Design review of the part built by this model. Coordinates are the model's own, in mm. A direction names the side the tool comes from. Coordinates: 2 decimals unless noted, no trailing zeros. Loops run counter-clockwise (first coordinate to the right, second up) from the corner with the lowest first, then second, coordinate; pieces in that order, holes last.
from build123d import *

# Parameters (mm, degrees)
SKETCH1_W           = 66
SKETCH1_H           = 95
SKETCH1_R           = 20
BOSS_EXTRUDE1_DEPTH = 12
BOSS_EXTRUDE3_DEPTH = 12
SKETCH6_R           = 6
CUT_EXTRUDE2_DEPTH  = 6
CHAMFER1_SIZE       = 20
CUT_EXTRUDE3_REACH  = 91.828
SKETCH7_R           = 3
SKETCH7_R_2         = 5
SKETCH9_R           = 3
CUT_EXTRUDE5_DEPTH  = 25
CUT_EXTRUDE6_REACH  = 91.828
SKETCH10_R          = 2.5
CUT_EXTRUDE7_DEPTH  = 4


with BuildPart() as part:
    # Sketch1 → Boss-Extrude1 (new body)
    with BuildSketch(Plane(origin=(0, 0, 0), x_dir=(1, 0, 0), z_dir=(0, 1, 0))):
        with Locations((0, -22.5)):
            Rectangle(SKETCH1_W, SKETCH1_H)
        with Locations(Location((0, -30, 0), (0, 0, 270))):
            Circle(SKETCH1_R, mode=Mode.SUBTRACT)
    extrude(amount=BOSS_EXTRUDE1_DEPTH)

    # Sketch3 → Boss-Extrude3 (add)
    with BuildSketch(Plane(origin=(0, 12, 0), x_dir=(1, 0, 0), z_dir=(0, 1, 0))):
        Polygon((55, 7), (43, 7), (43, -11), (55, -11), (55, -70), (33, -70), (33, 25), (55, 25), align=None)
    boss_extrude3 = extrude(amount=-BOSS_EXTRUDE3_DEPTH)

    # Mirror1: Boss-Extrude3 across plane
    add(boss_extrude3.mirror(Plane(origin=(0, 0, 0), x_dir=(0, 0, 1), z_dir=(1, 0, 0))))

    # Sketch6 → Cut-Extrude2 (cut)
    with BuildSketch(Plane(origin=(0, 12, 0), x_dir=(1, 0, 0), z_dir=(0, 1, 0))):
        with Locations(Location((-28, -51, 0), (0, 0, 270))):
            Circle(SKETCH6_R)
        with Locations(Location((28, -51, 0), (0, 0, 270))):
            Circle(SKETCH6_R)
    extrude(amount=-CUT_EXTRUDE2_DEPTH, mode=Mode.SUBTRACT)

    # Chamfer1
    chamfer1_edges = [part.edges().sort_by_distance(p)[0] for p in [
        (55, 6, 70),
        (-55, 6, 70),
    ]]
    chamfer(chamfer1_edges, length=CHAMFER1_SIZE)

    # Sketch7 → Cut-Extrude3 (cut, up to next)
    with BuildSketch(Plane(origin=(0, 12, 0), x_dir=(1, 0, 0), z_dir=(0, 1, 0)), mode=Mode.PRIVATE) as cut_extrude3_sk1:
        with Locations(Location((-49, 16, 0), (0, 0, 270))):
            Circle(SKETCH7_R)
    cut_extrude3_tool1 = extrude(cut_extrude3_sk1.sketch, amount=-CUT_EXTRUDE3_REACH, mode=Mode.PRIVATE) & part.part
    # Sketch7 → Cut-Extrude3 (cut, up to next)
    with BuildSketch(Plane(origin=(0, 12, 0), x_dir=(1, 0, 0), z_dir=(0, 1, 0)), mode=Mode.PRIVATE) as cut_extrude3_sk2:
        with Locations(Location((-49, -20, 0), (0, 0, 270))):
            Circle(SKETCH7_R)
    cut_extrude3_tool2 = extrude(cut_extrude3_sk2.sketch, amount=-CUT_EXTRUDE3_REACH, mode=Mode.PRIVATE) & part.part
    # Sketch7 → Cut-Extrude3 (cut, up to next)
    with BuildSketch(Plane(origin=(0, 12, 0), x_dir=(1, 0, 0), z_dir=(0, 1, 0)), mode=Mode.PRIVATE) as cut_extrude3_sk3:
        with Locations(Location((-25, -2, 0), (0, 0, 270))):
            Circle(SKETCH7_R_2)
    cut_extrude3_tool3 = extrude(cut_extrude3_sk3.sketch, amount=-CUT_EXTRUDE3_REACH, mode=Mode.PRIVATE) & part.part
    cut_extrude3_1 = cut_extrude3_tool1.solids().sort_by_distance((-49, 12, -16))[0]
    add(cut_extrude3_1, mode=Mode.SUBTRACT)
    cut_extrude3_2 = cut_extrude3_tool2.solids().sort_by_distance((-49, 12, 20))[0]
    add(cut_extrude3_2, mode=Mode.SUBTRACT)
    cut_extrude3_3 = cut_extrude3_tool3.solids().sort_by_distance((-25, 12, 2))[0]
    add(cut_extrude3_3, mode=Mode.SUBTRACT)
    cut_extrude3 = cut_extrude3_1 + cut_extrude3_2 + cut_extrude3_3  # Cut-Extrude3 as one shape, for the pattern or mirror that repeats it

    # Sketch9 → Cut-Extrude5 (cut)
    with BuildSketch(Plane.ZY.offset(43)):
        with Locations((2, 6)):
            Circle(SKETCH9_R)
    cut_extrude5 = extrude(amount=-CUT_EXTRUDE5_DEPTH, mode=Mode.SUBTRACT)

    # Mirror2: Cut-Extrude3, Cut-Extrude5 across plane
    add(cut_extrude3.mirror(Plane(origin=(0, 0, 0), x_dir=(0, 0, 1), z_dir=(1, 0, 0))), mode=Mode.SUBTRACT)
    add(cut_extrude5.mirror(Plane(origin=(0, 0, 0), x_dir=(0, 0, 1), z_dir=(1, 0, 0))), mode=Mode.SUBTRACT)

    # Sketch10 → Cut-Extrude6 (cut, up to next)
    with BuildSketch(Plane.XZ, mode=Mode.PRIVATE) as cut_extrude6_sk1:
        with Locations(Location((0, 63.234018716, 0), (0, 0, 270))):
            Circle(SKETCH10_R)
    cut_extrude6_tool1 = extrude(cut_extrude6_sk1.sketch, amount=-CUT_EXTRUDE6_REACH, mode=Mode.PRIVATE) & part.part
    # Sketch10 → Cut-Extrude6 (cut, up to next)
    with BuildSketch(Plane.XZ, mode=Mode.PRIVATE) as cut_extrude6_sk2:
        with Locations(Location((-33.234018716, 30, 0), (0, 0, 270))):
            Circle(SKETCH10_R)
    cut_extrude6_tool2 = extrude(cut_extrude6_sk2.sketch, amount=-CUT_EXTRUDE6_REACH, mode=Mode.PRIVATE) & part.part
    # Sketch10 → Cut-Extrude6 (cut, up to next)
    with BuildSketch(Plane.XZ, mode=Mode.PRIVATE) as cut_extrude6_sk3:
        with Locations(Location((0, -3.234018716, 0), (0, 0, 270))):
            Circle(SKETCH10_R)
    cut_extrude6_tool3 = extrude(cut_extrude6_sk3.sketch, amount=-CUT_EXTRUDE6_REACH, mode=Mode.PRIVATE) & part.part
    # Sketch10 → Cut-Extrude6 (cut, up to next)
    with BuildSketch(Plane.XZ, mode=Mode.PRIVATE) as cut_extrude6_sk4:
        with Locations(Location((33.234018716, 30, 0), (0, 0, 270))):
            Circle(SKETCH10_R)
    cut_extrude6_tool4 = extrude(cut_extrude6_sk4.sketch, amount=-CUT_EXTRUDE6_REACH, mode=Mode.PRIVATE) & part.part
    add(cut_extrude6_tool1.solids().sort_by_distance((0, 0, 63.234019))[0], mode=Mode.SUBTRACT)
    add(cut_extrude6_tool2.solids().sort_by_distance((-33.234019, 0, 30))[0], mode=Mode.SUBTRACT)
    add(cut_extrude6_tool3.solids().sort_by_distance((0, 0, -3.234019))[0], mode=Mode.SUBTRACT)
    add(cut_extrude6_tool4.solids().sort_by_distance((33.234019, 0, 30))[0], mode=Mode.SUBTRACT)

    # Sketch12 → Cut-Extrude7 (cut)
    with BuildSketch(Plane(origin=(0, 12, 0), x_dir=(1, 0, 0), z_dir=(0, 1, 0))):
        Polygon((3.334261142, -59.954887332), (-1.17268051, -58.706898172), (-4.506941652, -61.986029556), (-3.334261142, -66.5131501), (1.17268051, -67.76113926), (4.506941652, -64.482007876), align=None)
        Polygon((-29.899757573, -33.279131384), (-28.727077064, -28.75201084), (-32.061338206, -25.472879456), (-36.568279858, -26.720868616), (-37.740960368, -31.24798916), (-34.406699225, -34.527120544), align=None)
        Polygon((-3.282764492, -0.096665492), (1.24307489, -1.274280833), (4.525839382, 2.056403375), (3.282764492, 6.564702924), (-1.24307489, 7.742318264), (-4.525839382, 4.411634056), align=None)
        Polygon((29.951254224, -26.669315792), (28.708179334, -31.177615341), (31.990943826, -34.508299548), (36.516783208, -33.330684208), (37.759858098, -28.822384659), (34.477093606, -25.491700452), align=None)
    extrude(amount=-CUT_EXTRUDE7_DEPTH, mode=Mode.SUBTRACT)


solid = part.part
Q1. The part is to be moulded in two halves that separate along Y. For faces 4 (the flat face through (1, 6, -25)), 5 (the cylindrical face through (-19.19, 4.85, 4.77)), 6 (the flat face through (-2, 8, 65)), 7 (the flat face through (18, 6, 2)), say which applies: pulls with the +Y half, pulls with the -Y half, needs draft (parallel to the pull), parting line crosses it, or undercut.
Q2. Take a section at B-B, the plane x = 49. Write out the cut boundary in (y, z), then the cut area to 3 significant figures.
Q3. Take a section at D-D, the plane y = 10.25. Give the number of separate pieces and of enclosed holes in the cut face, then the cut area to 3 significant figures.
Q4. Take a section at A-A, the plane z = -16. Write out the cut boundary in (x, y).
Q5. Machinability: for faces 1 (the flat face through (55, 6, 30)), 2 (the flat face through (-32.18, 10.03, 33.91)), 3 (the flat face through (43, 9, 0)), which of the approach directions +Z, -Z, +X, -X, +Y, -Y give a long, thin tool a straight path to every point of the face, cutting with its end or side? Answer none if there is none.
Q6. For line 1 (X direction, y = 6.75, z = 30); line 2 (X direction, y = 8, z = 55); line 3 (X direction, y = 8, z = -13.5), list the stretches that pass through material, from the lowest coordinate up.
Q7. Take a section at C-C, the plane z = 36.5. Write out the cut boundary in (x, y).
Q8. Clearance check with flat-ended pins moving along their axes: pin 1 Ø5 at (y, z) = (6, 2) entering from -X; pin 2 Ø6 at (x, z) = (29, 53.5) entering from +Y; pin 3 Ø6 at (x, y) = (-40.5, 5) entering from +Z. State where each tip first meets the part, or that it passes through.
Entries:
1. face 4: needs draft
1. face 5: undercut
1. face 6: pulls with the +Y half
1. face 7: undercut
2. outline: (0, -25) - (12, -25) - (12, -19) - (0, -19) - close; (0, -13) - (12, -13) - (12, -7) - (0, -7) - close; (0, 11) - (12, 11) - (12, 17) - (0, 17) - close; (0, 23) - (12, 23) - (12, 56) - (0, 56) - close
2. area: 612 mm2
3. separate pieces: 1
3. enclosed holes: 13
3. area: 7,640 mm2
4. outline: (-55, 0) - (-52, 0) - (-52, 12) - (-55, 12) - close; (-46, 0) - (46, 0) - (46, 12) - (-46, 12) - close; (52, 0) - (55, 0) - (55, 12) - (52, 12) - close
5. face 1: +Z, -Z, +X, +Y, -Y
5. face 2: +Y
5. face 3: +X, +Y, -Y
6. line 1: x = -55 to -35.73, -30.73 to -20, 20 to 30.73, 35.73 to 55
6. line 2: x = -50 to -32.47, -23.53 to 23.53, 32.47 to 50
6. line 3: x = -55 to -50.66, -47.34 to 47.34, 50.66 to 55
7. outline: (-55, 0) - (-18.91, 0) - (-18.91, 12) - (-55, 12) - close; (18.91, 0) - (55, 0) - (55, 12) - (18.91, 12) - close
8. pin 1: stops at x = -18
8. pin 2: stops at y = 6
8. pin 3: stops at z = 67.5
